```python
from build123d import *

# Parameters (mm, degrees)
FILLET1_R               = 1.5
SKETCH4_W               = 2.5
SKETCH4_H               = 4.5
SKETCH4_W_2             = 8
SKETCH4_H_2             = 3.5
CUT_EXTRUDE1_DEPTH      = 3.5
SKETCH3_W               = 7.5
SKETCH3_H               = 6
CUT_EXTRUDE2_DEPTH      = 12.470832747
CUT_EXTRUDE5_DEPTH      = 11.900917559
CUT_EXTRUDE5_DEPTH_BACK = 1
SKETCH5_R               = 2
CUT_EXTRUDE6_START      = -0.5
CUT_EXTRUDE6_DEPTH      = 1.5
SKETCH9_W               = 1
SKETCH9_H               = 3
CUT_EXTRUDE9_DEPTH      = 12.470832747
CUT_EXTRUDE10_DEPTH     = 0.7
CUT_EXTRUDE11_DEPTH     = 0.7
CUT_EXTRUDE12_DEPTH     = 4
BOSS_EXTRUDE1_DEPTH     = 2
BOSS_EXTRUDE2_DEPTH     = 2
CUT_EXTRUDE17_DEPTH     = 0.45
CUT_EXTRUDE18_DEPTH     = 0.45
CUT_EXTRUDE19_DEPTH     = 0.5
CUT_EXTRUDE20_DEPTH     = 0.5
CUT_EXTRUDE22_START     = -3.5
SKETCH29_W              = 8.5
SKETCH29_H              = 3.5
CUT_EXTRUDE22_DEPTH     = 3.5
BOSS_EXTRUDE6_DEPTH     = 0.5
SKETCH33_W              = 2.25
SKETCH33_H              = 0.2
CUT_EXTRUDE23_DEPTH     = 1.5
SKETCH35_W              = 6.5
SKETCH35_H              = 2.080921332
CUT_EXTRUDE24_DEPTH     = 1
CUT_EXTRUDE25_DEPTH     = 11.750814086
SKETCH37_W              = 1.75
SKETCH37_H              = 0.2
CUT_EXTRUDE26_DEPTH     = 4.5
SKETCH38_W              = 2.5
SKETCH38_H              = 0.2
CUT_EXTRUDE27_DEPTH     = 12.470832747
SKETCH39_W              = 1
SKETCH39_H              = 2.5
BOSS_EXTRUDE9_DEPTH     = 2
SKETCH40_W              = 1.5
SKETCH40_H              = 2.5
BOSS_EXTRUDE10_DEPTH    = 2.5
CUT_EXTRUDE28_DEPTH     = 16.808225868
FILLET3_R               = 0.1


with BuildPart() as part:
    # Sketch1 → Loft1 section 0
    with BuildSketch(Plane(origin=(0, 0, 0), x_dir=(1, 0, 0), z_dir=(0, 1, 0))):
        with BuildLine():
            Line((-7.3, 7.3), (7.3, 7.3))
            Line((7.3, 7.3), (7.3, -7.3))
            Line((7.3, -7.3), (-7.3, -7.3))
            Line((-7.3, -7.3), (-7.3, 7.3))
        make_face()
    # Sketch2 → Loft1 section 1
    with BuildSketch(Plane(origin=(0, 5, 0), x_dir=(1, 0, 0), z_dir=(0, 1, 0))):
        with BuildLine():
            Line((-5.5, 6.5), (5.5, 6.5))
            Line((5.5, 6.5), (5.5, -4.5))
            Line((5.5, -4.5), (-5.5, -4.5))
            Line((-5.5, -4.5), (-5.5, 6.5))
        make_face()
    loft()

    # Fillet1
    fillet1_edges = [part.edges().sort_by_distance(p)[0] for p in [
        (0, 5, -6.5),
    ]]
    fillet(fillet1_edges, radius=FILLET1_R)

    # Sketch4 → Cut-Extrude1 (cut)
    with BuildSketch(Plane(origin=(0, 5, 0), x_dir=(1, 0, 0), z_dir=(0, 1, 0))):
        with Locations((-6.05, -5.05)):
            Rectangle(SKETCH4_W, SKETCH4_H)
        with Locations((6.05, 5.05)):
            Rectangle(SKETCH4_W, SKETCH4_H)
        with Locations((-6.05, 5.05)):
            Rectangle(SKETCH4_W, SKETCH4_H)
        with Locations((6.05, -5.05)):
            Rectangle(SKETCH4_W, SKETCH4_H)
        with Locations((0, -5.55)):
            Rectangle(SKETCH4_W_2, SKETCH4_H_2)
    extrude(amount=-CUT_EXTRUDE1_DEPTH, mode=Mode.SUBTRACT)

    # Shell2: read off the stored shape, not the designer's step
    # Shell2: loft between two sections, ruled curve by curve
    shell2_from = [
        Edge.make_line((5.705760369, 0, 1.3), (5.705760369, 0, -1.3)),
        Edge.make_line((-3.3, 0, -5.780921332), (3.3, 0, -5.780921332)),
        Edge.make_line((-5.705760369, 0, 1.3), (-5.705760369, 0, -1.3)),
        Edge.make_line((5.705760369, 0, -1.3), (3.3, 0, -1.3)),
        Edge.make_line((-5.705760369, 0, -1.3), (-3.3, 0, -1.3)),
        Edge.make_line((3.3, 0, -5.780921332), (3.3, 0, -1.3)),
        Edge.make_line((3.3, 0, 1.3), (3.3, 0, 2.3)),
        Edge.make_line((-3.3, 0, -5.780921332), (-3.3, 0, -1.3)),
        Edge.make_line((-3.3, 0, 2.3), (-3.3, 0, 1.3)),
        Edge.make_line((-3.3, 0, 1.3), (-5.705760369, 0, 1.3)),
        Edge.make_line((5.705760369, 0, 1.3), (3.3, 0, 1.3)),
        Edge.make_line((3.3, 0, 2.3), (-3.3, 0, 2.3)),
    ]
    shell2_to = [
        Edge.make_line((4.445760369, 3.5, 1.3), (4.445760369, 3.5, -1.3)),
        Edge.make_line((-3.3, 3.5, -5.220921332), (3.3, 3.5, -5.220921332)),
        Edge.make_line((-4.445760369, 3.5, 1.3), (-4.445760369, 3.5, -1.3)),
        Edge.make_line((4.445760369, 3.5, -1.3), (3.3, 3.5, -1.3)),
        Edge.make_line((-4.445760369, 3.5, -1.3), (-3.3, 3.5, -1.3)),
        Edge.make_line((3.3, 3.5, -5.220921332), (3.3, 3.5, -1.3)),
        Edge.make_line((3.3, 3.5, 1.3), (3.3, 3.5, 2.3)),
        Edge.make_line((-3.3, 3.5, -5.220921332), (-3.3, 3.5, -1.3)),
        Edge.make_line((-3.3, 3.5, 2.3), (-3.3, 3.5, 1.3)),
        Edge.make_line((-3.3, 3.5, 1.3), (-4.445760369, 3.5, 1.3)),
        Edge.make_line((4.445760369, 3.5, 1.3), (3.3, 3.5, 1.3)),
        Edge.make_line((3.3, 3.5, 2.3), (-3.3, 3.5, 2.3)),
    ]
    shell2 = Solid(Shell([*[Face.make_surface_from_curves(shell2_from[k], shell2_to[k]) for k in range(12)], Face(Wire(shell2_from)), Face(Wire(shell2_to))]))
    add(shell2, mode=Mode.SUBTRACT)

    # Sketch3 → Cut-Extrude2 (cut, through all)
    with BuildSketch(Plane.XZ):
        Rectangle(SKETCH3_W, SKETCH3_H)
    extrude(amount=-CUT_EXTRUDE2_DEPTH, mode=Mode.SUBTRACT)

    # Sketch5 → Cut-Extrude5 (cut, two sides: drawn at the far end of the back side and taken through both)
    with BuildSketch(Plane(origin=(0, 1.5, 0), x_dir=(1, 0, 0), z_dir=(0, 1, 0)).offset(-CUT_EXTRUDE5_DEPTH_BACK)):
        with Locations((0, -5.3)):
            Circle(SKETCH5_R)
    extrude(amount=CUT_EXTRUDE5_DEPTH + CUT_EXTRUDE5_DEPTH_BACK, mode=Mode.SUBTRACT)

    # Cut-Extrude6: read off the stored shape, not the designer's step
    # Cut-Extrude6 outline → Cut-Extrude6 (cut)
    with BuildSketch(Plane.XZ.offset(CUT_EXTRUDE6_START)):
        with BuildLine():
            Line((1.936491673, 5.8), (-1.936491673, 5.8))
            ThreePointArc((-1.936491673, 5.8), (-2, 5.3), (-1.936491673, 4.8))
            Line((-1.936491673, 4.8), (1.936491673, 4.8))
            ThreePointArc((1.936491673, 4.8), (2, 5.3), (1.936491673, 5.8))
        make_face()
    extrude(amount=CUT_EXTRUDE6_DEPTH, mode=Mode.SUBTRACT)

    # Sketch9 → Cut-Extrude9 (cut, through all)
    with BuildSketch(Plane(origin=(0, 0, 0), x_dir=(1, 0, 0), z_dir=(0, 1, 0))):
        with Locations((-5.3, 4.3)):
            Rectangle(SKETCH9_W, SKETCH9_H)
        with Locations((5.3, 4.3)):
            Rectangle(SKETCH9_W, SKETCH9_H)
        with Locations((-5.3, -4.3)):
            Rectangle(SKETCH9_W, SKETCH9_H)
        with Locations((5.3, -4.3)):
            Rectangle(SKETCH9_W, SKETCH9_H)
    extrude(amount=CUT_EXTRUDE9_DEPTH, mode=Mode.SUBTRACT)

    # Sketch11 → Cut-Extrude10 (cut)
    with BuildSketch(Plane(origin=(0, 0, 1.3), x_dir=(-1, 0, 0), z_dir=(0, 0, -1))):
        Polygon((-3.75, 0), (-5.705760369, 0), (-4.445760369, 3.5), (-3.75, 3.5), align=None)
        Polygon((3.75, 0), (3.75, 3.5), (4.445760369, 3.5), (5.705760369, 0), align=None)
    extrude(amount=-CUT_EXTRUDE10_DEPTH, mode=Mode.SUBTRACT)

    # Sketch12 → Cut-Extrude11 (cut)
    with BuildSketch(Plane.XY.offset(-1.3)):
        Polygon((3.75, 0), (5.705760369, 0), (4.445760369, 3.5), (3.75, 3.5), align=None)
        Polygon((-3.75, 0), (-5.705760369, 0), (-4.445760369, 3.5), (-3.75, 3.5), align=None)
    extrude(amount=-CUT_EXTRUDE11_DEPTH, mode=Mode.SUBTRACT)

    # Sketch13 → Cut-Extrude12 (cut)
    with BuildSketch(Plane(origin=(0, 0, 2), x_dir=(-1, 0, 0), z_dir=(0, 0, -1))):
        Polygon((3.75, 3.5), (5.25, 3.5), (5.705760369, 0), (3.75, 0), align=None)
        Polygon((-3.75, 3.5), (-5.25, 3.5), (-5.705760369, 0), (-3.75, 0), align=None)
    extrude(amount=CUT_EXTRUDE12_DEPTH, mode=Mode.SUBTRACT)

    # Sketch14 → Boss-Extrude1 (add)
    with BuildSketch(Plane(origin=(-3.75, 0, 0), x_dir=(0, 0, -1), z_dir=(1, 0, 0))):
        Polygon((-2, 3.5), (-1.5, 3.5), (-2, 3), align=None)
        Polygon((1.5, 3.5), (2, 3.5), (2, 3), align=None)
    extrude(amount=-BOSS_EXTRUDE1_DEPTH)

    # Sketch15 → Boss-Extrude2 (add)
    with BuildSketch(Plane.ZY.offset(-3.75)):
        Polygon((2, 3.5), (2, 3), (1.5, 3.5), align=None)
        Polygon((-2, 3.5), (-2, 3), (-1.5, 3.5), align=None)
    extrude(amount=-BOSS_EXTRUDE2_DEPTH)

    # Sketch18 → Cut-Extrude17 (cut)
    with BuildSketch(Plane(origin=(-3.3, 0, 0), x_dir=(0, 0, -1), z_dir=(1, 0, 0))):
        Polygon((5.220921332, 3.5), (3, 3.5), (3, 0), (5.780921332, 0), align=None)
    extrude(amount=-CUT_EXTRUDE17_DEPTH, mode=Mode.SUBTRACT)

    # Sketch19 → Cut-Extrude18 (cut)
    with BuildSketch(Plane.ZY.offset(-3.3)):
        Polygon((-5.780921332, 0), (-3, 0), (-3, 3.5), (-5.220921332, 3.5), align=None)
    extrude(amount=-CUT_EXTRUDE18_DEPTH, mode=Mode.SUBTRACT)

    # Sketch22 → Cut-Extrude19 (cut)
    with BuildSketch(Plane(origin=(-3.75, 0, 0), x_dir=(0, 0, -1), z_dir=(1, 0, 0))):
        Polygon((5.780921332, 0), (2.280921332, 0), (2.280921332, 3.5), (5.220921332, 3.5), align=None)
    extrude(amount=-CUT_EXTRUDE19_DEPTH, mode=Mode.SUBTRACT)

    # Sketch23 → Cut-Extrude20 (cut)
    with BuildSketch(Plane.ZY.offset(-3.75)):
        Polygon((-5.780921332, 0), (-2.280921332, 0), (-2.280921332, 3.5), (-5.220921332, 3.5), align=None)
    extrude(amount=-CUT_EXTRUDE20_DEPTH, mode=Mode.SUBTRACT)

    # Sketch29 → Cut-Extrude22 (cut)
    with BuildSketch(Plane.XZ.offset(CUT_EXTRUDE22_START)):
        with Locations((0, -4.030921332)):
            Rectangle(SKETCH29_W, SKETCH29_H)
    extrude(amount=CUT_EXTRUDE22_DEPTH, mode=Mode.SUBTRACT)

    # Sketch31 → Boss-Extrude6 (add)
    with BuildSketch(Plane.XZ.offset(-3.5)):
        Polygon((-4.25, -3), (-4.25, -5.780921332), (-3.25, -5.780921332), (-3.25, -3.7), (3.25, -3.7), (3.25, -5.780921332), (4.25, -5.780921332), (4.25, -3), (3.75, -3), (-3.75, -3), align=None)
    extrude(amount=BOSS_EXTRUDE6_DEPTH)

    # Sketch33 → Cut-Extrude23 (cut)
    with BuildSketch(Plane.XZ.offset(-3)):
        with Locations((-3.125, -3.1)):
            Rectangle(SKETCH33_W, SKETCH33_H)
        with Locations((3.125, -3.1)):
            Rectangle(SKETCH33_W, SKETCH33_H)
    extrude(amount=-CUT_EXTRUDE23_DEPTH, mode=Mode.SUBTRACT)

    # Sketch35 → Cut-Extrude24 (cut)
    with BuildSketch(Plane.XZ.offset(-3.5)):
        with Locations((0, -4.740460666)):
            Rectangle(SKETCH35_W, SKETCH35_H)
    extrude(amount=-CUT_EXTRUDE24_DEPTH, mode=Mode.SUBTRACT)

    # Sketch36 → Cut-Extrude25 (cut, through all)
    with BuildSketch(Plane.XZ.offset(-3)):
        with BuildLine():
            Line((-1.490805152, -3), (1.490805152, -3))
            ThreePointArc((1.490805152, -3), (0, -3.35), (-1.490805152, -3))
        make_face()
    extrude(amount=-CUT_EXTRUDE25_DEPTH, mode=Mode.SUBTRACT)

    # Sketch37 → Cut-Extrude26 (cut)
    with BuildSketch(Plane.XZ):
        with Locations((-2.875, 3.1)):
            Rectangle(SKETCH37_W, SKETCH37_H)
        with Locations((2.875, 3.1)):
            Rectangle(SKETCH37_W, SKETCH37_H)
    extrude(amount=-CUT_EXTRUDE26_DEPTH, mode=Mode.SUBTRACT)

    # Sketch38 → Cut-Extrude27 (cut, through all)
    with BuildSketch(Plane.XZ):
        with Locations((0, 3.1)):
            Rectangle(SKETCH38_W, SKETCH38_H)
    extrude(amount=-CUT_EXTRUDE27_DEPTH, mode=Mode.SUBTRACT)

    # Sketch39 → Boss-Extrude9 (add)
    with BuildSketch(Plane.XZ):
        with Locations((-6.3, 4.55)):
            Rectangle(SKETCH39_W, SKETCH39_H)
        with Locations((-6.3, -4.55)):
            Rectangle(SKETCH39_W, SKETCH39_H)
        with Locations((6.3, 4.55)):
            Rectangle(SKETCH39_W, SKETCH39_H)
        with Locations((6.3, -4.55)):
            Rectangle(SKETCH39_W, SKETCH39_H)
    extrude(amount=BOSS_EXTRUDE9_DEPTH)

    # Sketch40 → Boss-Extrude10 (add)
    with BuildSketch(Plane.XZ.offset(2)):
        with Locations((-6.05, 4.55)):
            Rectangle(SKETCH40_W, SKETCH40_H)
        with Locations((-6.05, -4.55)):
            Rectangle(SKETCH40_W, SKETCH40_H)
        with Locations((6.05, 4.55)):
            Rectangle(SKETCH40_W, SKETCH40_H)
        with Locations((6.05, -4.55)):
            Rectangle(SKETCH40_W, SKETCH40_H)
    extrude(amount=BOSS_EXTRUDE10_DEPTH)

    # Sketch41 → Cut-Extrude28 (cut, through all)
    with BuildSketch(Plane.XY.offset(5.8)):
        Polygon((-6.05, -4.5), (-6.8, -2), (-6.8, -4.5), align=None)
        Polygon((-5.3, -3), (-6.05, -4.5), (-5.3, -4.5), align=None)
        Polygon((5.3, -4.5), (6.05, -4.5), (5.3, -3), align=None)
        Polygon((6.8, -4.5), (6.8, -2), (6.05, -4.5), align=None)
    extrude(amount=-CUT_EXTRUDE28_DEPTH, mode=Mode.SUBTRACT)

    # Fillet3
    fillet3_edges = [part.edges().sort_by_distance(p)[0] for p in [
        (6.05, -4.5, -4.55),
        (-6.05, -4.5, -4.55),
        (-6.05, -4.5, 4.55),
        (6.05, -4.5, 4.55),
    ]]
    fillet(fillet3_edges, radius=FILLET3_R)


solid = part.part
```
Can you work these out from the model? Positions are in its coordinate system, mm. A direction names the side the tool comes from. Round coordinates to 2 decimals unless told otherwise and drop trailing zeros. Loops run counter-clockwise (first coordinate to the right, second up) from the corner with the lowest first, then second, coordinate; pieces in that order, holes last. Notation, with made-up numbers: M -24,30 L 17,30 A24 cw 17,47 Z; hole C 25,41.5 d4. An arc over 180 degrees is marked long. Answer as a JSON object with one key per item and string values. Group by question number.
Q1. Will these pins go through, and if not, where does the flat tip stop? pin 1 (1 mm diameter, centred on x = -5.5, z = 4.5, fed in from +Y); pin 2 (0.9 mm diameter, centred on y = -0.5, z = 4.5, fed in from -X); pin 3 (1.3 mm diameter, centred on x = 0.5, y = 2, fed in from +Z).
Q2. Imagine slicing it at B-B, the plane x = 5. Count the separate pieces of the cut face and the enclosed holes in it, then the cut area to 3 significant figures.
Q3. Imagine slicing it at A-A, the plane y = -0.5. Please give me the cut outline in (x, z).
Q4. Please list where these lines run through material, in increasing order: L1, parallel to X at y = 3.1, z = 5.3; L2, parallel to X at y = 1, z = -3.75; L3, parallel to Y at x = -6.25, z = -6.5.
Q5. On a 3-axis mill with a long thin cutter (end or side, diameter ignored), from which of +Z, -Z, +X, -X, +Y, -Y can I reach the whole of each face in a straight line? I mean faces 1 (the flat face through (6, 2, 2.8)), 2 (the flat face through (3.25, 4, -5)), 3 (the flat face through (-6, -2, -5.8)). Say none if no direction works.
Findings:
{
 "1": {"pin 1": "stops at y = 1.5", "pin 2": "stops at x = -6.8", "pin 3": "stops at z = 3.66"},
 "2": {"separate pieces": "3", "enclosed holes": "0", "area": "17.9 mm2"},
 "3": {"outline": "M -6.8,-5.8 L -5.8,-5.8 L -5.8,-3.3 L -6.8,-3.3 Z; M -6.8,3.3 L -5.8,3.3 L -5.8,5.8 L -6.8,5.8 Z; M 5.8,-5.8 L 6.8,-5.8 L 6.8,-3.3 L 5.8,-3.3 Z; M 5.8,3.3 L 6.8,3.3 L 6.8,5.8 L 5.8,5.8 Z"},
 "4": {"L1": "x = -4.8 to -4, 4 to 4.8", "L2": "x = -6.94 to -5.8, -4.8 to -4.25, 4.25 to 4.8, 5.8 to 6.94", "L3": "y = 0 to 1.5"},
 "5": {"face 1": "+Y", "face 2": "-Y", "face 3": "-Z, +X, -X, -Y"}
}
